CAD build for the part. Positions are in the model's coordinates, mm. Face numbers are marked on the shaded views. Round coordinates to 2 decimals unless told otherwise and drop trailing zeros. Loops run counter-clockwise (first coordinate to the right, second up) from the corner with the lowest first, then second, coordinate; pieces in that order, holes last.
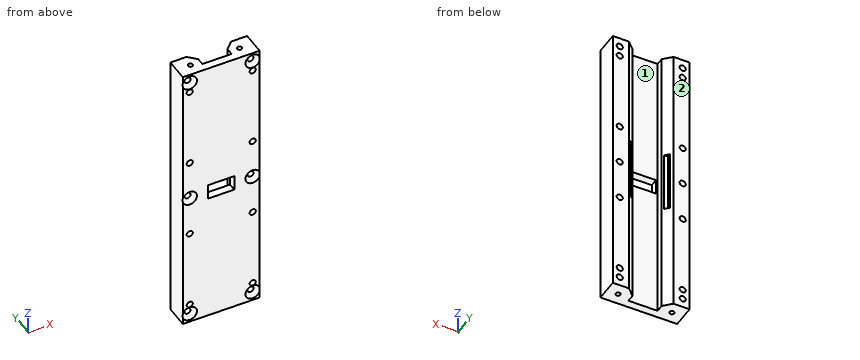
```python
from build123d import *

# Parameters (mm, degrees)
BOSS_EXTRU_1_DEPTH       = 184
ESQUISSE2_R              = 2
ENL_V_MAT_EXTRU_1_DEPTH  = 205.56
ESQUISSE4_R              = 2
ENL_V_MAT_EXTRU_2_DEPTH  = 205.56
CHANFREIN1_SIZE          = 2.7
ESQUISSE6_W              = 26
ESQUISSE6_H              = 40
ENL_V_MAT_EXTRU_3_DEPTH  = 4
ESQUISSE8_W              = 17
ESQUISSE8_H              = 10
ENL_V_MAT_EXTRU_6_DEPTH  = 10
ESQUISSE7_R              = 1.5
ENL_V_MAT_EXTRU_5_DEPTH  = 5
ESQUISSE9_R              = 1.5
ENL_V_MAT_EXTRU_10_DEPTH = 5


with BuildPart() as part:
    # Esquisse1 → Boss.-Extru.1 (new body)
    with BuildSketch(Plane.XY):
        Polygon((0, 0), (50, 0), (50, 15), (39.5, 15), (34.5, 10), (34.5, 5.083005244), (15.5, 5.083005244), (15.5, 10), (10.5, 15), (0, 15), align=None)
    extrude(amount=BOSS_EXTRU_1_DEPTH)

    # Esquisse2 → Enlèv. mat.-Extru.1 (cut)
    with BuildSketch(Plane(origin=(0, 15, 0), x_dir=(-1, 0, 0), z_dir=(0, 1, 0))):
        with Locations(Location((-4.5, 12.78, 0), (0, 0, 90))):
            Circle(ESQUISSE2_R)
        with Locations(Location((-45.5, 12.78, 0), (0, 0, 90))):
            Circle(ESQUISSE2_R)
        with Locations(Location((-4.5, 65.52, 0), (0, 0, 90))):
            Circle(ESQUISSE2_R)
        with Locations(Location((-45.5, 65.52, 0), (0, 0, 90))):
            Circle(ESQUISSE2_R)
        with Locations(Location((-4.5, 118.26, 0), (0, 0, 90))):
            Circle(ESQUISSE2_R)
        with Locations(Location((-45.5, 118.26, 0), (0, 0, 90))):
            Circle(ESQUISSE2_R)
        with Locations(Location((-4.5, 171, 0), (0, 0, 90))):
            Circle(ESQUISSE2_R)
        with Locations(Location((-45.5, 171, 0), (0, 0, 90))):
            Circle(ESQUISSE2_R)
    extrude(amount=-ENL_V_MAT_EXTRU_1_DEPTH, mode=Mode.SUBTRACT)

    # Esquisse4 → Enlèv. mat.-Extru.2 (cut)
    with BuildSketch(Plane(origin=(0, 15, 0), x_dir=(-1, 0, 0), z_dir=(0, 1, 0))):
        with Locations(Location((-4.5, 6, 0), (0, 0, 90))):
            Circle(ESQUISSE4_R)
        with Locations(Location((-45.5, 6, 0), (0, 0, 90))):
            Circle(ESQUISSE4_R)
        with Locations(Location((-45.5, 178, 0), (0, 0, 90))):
            Circle(ESQUISSE4_R)
        with Locations(Location((-4.5, 178, 0), (0, 0, 90))):
            Circle(ESQUISSE4_R)
        with Locations(Location((-4.5, 92, 0), (0, 0, 90))):
            Circle(ESQUISSE4_R)
        with Locations(Location((-45.5, 92, 0), (0, 0, 90))):
            Circle(ESQUISSE4_R)
    extrude(amount=-ENL_V_MAT_EXTRU_2_DEPTH, mode=Mode.SUBTRACT)

    # Chanfrein1
    # the kernel refuses this chamfer: 2.7 mm, written as the material it takes off along each edge
    with BuildSketch(Plane(origin=(4.5, 0, 6), x_dir=(0, 0, 1), z_dir=(-1, 0, 0))) as chanfrein1_piece_1:
        Polygon((2 + CHANFREIN1_SIZE, 0), (2, CHANFREIN1_SIZE), (2, 0), align=None)
    revolve(axis=Axis((4.5, 0, 6), (0, 1, 0)), mode=Mode.SUBTRACT)
    with BuildSketch(Plane(origin=(45.5, 0, 6), x_dir=(0, 0, 1), z_dir=(-1, 0, 0))) as chanfrein1_piece_2:
        Polygon((2 + CHANFREIN1_SIZE, 0), (2, CHANFREIN1_SIZE), (2, 0), align=None)
    revolve(axis=Axis((45.5, 0, 6), (0, 1, 0)), mode=Mode.SUBTRACT)
    with BuildSketch(Plane(origin=(45.5, 0, 178), x_dir=(0, 0, 1), z_dir=(-1, 0, 0))) as chanfrein1_piece_3:
        Polygon((2 + CHANFREIN1_SIZE, 0), (2, CHANFREIN1_SIZE), (2, 0), align=None)
    revolve(axis=Axis((45.5, 0, 178), (0, 1, 0)), mode=Mode.SUBTRACT)
    with BuildSketch(Plane(origin=(4.5, 0, 178), x_dir=(0, 0, 1), z_dir=(-1, 0, 0))) as chanfrein1_piece_4:
        Polygon((2 + CHANFREIN1_SIZE, 0), (2, CHANFREIN1_SIZE), (2, 0), align=None)
    revolve(axis=Axis((4.5, 0, 178), (0, 1, 0)), mode=Mode.SUBTRACT)
    with BuildSketch(Plane(origin=(4.5, 0, 92), x_dir=(0, 0, 1), z_dir=(-1, 0, 0))) as chanfrein1_piece_5:
        Polygon((2 + CHANFREIN1_SIZE, 0), (2, CHANFREIN1_SIZE), (2, 0), align=None)
    revolve(axis=Axis((4.5, 0, 92), (0, 1, 0)), mode=Mode.SUBTRACT)
    with BuildSketch(Plane(origin=(45.5, 0, 92), x_dir=(0, 0, 1), z_dir=(-1, 0, 0))) as chanfrein1_piece_6:
        Polygon((2 + CHANFREIN1_SIZE, 0), (2, CHANFREIN1_SIZE), (2, 0), align=None)
    revolve(axis=Axis((45.5, 0, 92), (0, 1, 0)), mode=Mode.SUBTRACT)

    # Esquisse6 → Enlèv. mat.-Extru.3 (cut)
    with BuildSketch(Plane(origin=(0, 15, 0), x_dir=(1, 0, 0), z_dir=(0, 1, 0))):
        with Locations((25, -92)):
            Rectangle(ESQUISSE6_W, ESQUISSE6_H)
    extrude(amount=-ENL_V_MAT_EXTRU_3_DEPTH, mode=Mode.SUBTRACT)

    # Esquisse8 → Enlèv. mat.-Extru.6 (cut)
    with BuildSketch(Plane(origin=(0, 5.083005244, 0), x_dir=(1, 0, 0), z_dir=(0, 1, 0))):
        with Locations((25, -92)):
            Rectangle(ESQUISSE8_W, ESQUISSE8_H)
    extrude(amount=-ENL_V_MAT_EXTRU_6_DEPTH, mode=Mode.SUBTRACT)

    # Esquisse7 → Enlèv. mat.-Extru.5 (cut)
    with BuildSketch(Plane.XY.offset(184)):
        with Locations((9, 7.5)):
            Circle(ESQUISSE7_R)
        with Locations((41, 7.5)):
            Circle(ESQUISSE7_R)
    extrude(amount=-ENL_V_MAT_EXTRU_5_DEPTH, mode=Mode.SUBTRACT)

    # Esquisse9 → Enlèv. mat.-Extru.10 (cut)
    with BuildSketch(Plane(origin=(0, 0, 0), x_dir=(-1, 0, 0), z_dir=(0, 0, -1))):
        with Locations((-42.5, 7.5)):
            Circle(ESQUISSE9_R)
        with Locations((-7.5, 7.5)):
            Circle(ESQUISSE9_R)
    extrude(amount=-ENL_V_MAT_EXTRU_10_DEPTH, mode=Mode.SUBTRACT)


solid = part.part
```
Item 1: Two-plate mould, pull along X, no slides. Class the marked faces 1 and 2: released by +X, released by -X, zero draft, split by the parting line, or undercut.
Answers follow:
face 1: undercut
face 2: zero draft
Item 2: Cut at A-A, the plane z = 12.78. Give the cut face in (x, y).
Answers follow:
outline: (0, 0) - (2.5, 0) - (2.5, 15) - (0, 15) - close; (6.5, 0) - (43.5, 0) - (43.5, 15) - (39.5, 15) - (34.5, 10) - (34.5, 5.08) - (15.5, 5.08) - (15.5, 10) - (10.5, 15) - (6.5, 15) - close; (47.5, 0) - (50, 0) - (50, 15) - (47.5, 15) - close
Item 3: Flat gauge pins, fed straight in: P1, Ø8, axis at y = 5, z = 81, coming from the -X side; P2, Ø1.2, axis at x = 12.5, z = 87.5, coming from the +Y side; P3, Ø6.5, axis at x = 45.5, z = 178, coming from the -Y side; P4, Ø1.4, axis at x = 43, y = 7.5, coming from the -Z side. Where does each tip first touch, or does it go through?
Answers follow:
P1: stops at x = 0
P2: stops at y = 13.6
P3: stops at y = 1.45
P4: stops at z = 5
Item 4: Cut at B-B, the plane z = 122. Give the cut face in (x, y).
Answers follow:
outline: (0, 0) - (50, 0) - (50, 15) - (39.5, 15) - (34.5, 10) - (34.5, 5.08) - (15.5, 5.08) - (15.5, 10) - (10.5, 15) - (0, 15) - close
Item 5: Probe line 1 (X direction, y = 8.5, z = 12.78); line 2 (X direction, y = 5, z = 13); line 3 (X direction, y = 7.25, z = 102.5). List the from-to ranges inside material, lowest first.
Answers follow:
line 1: x = 0 to 2.5, 6.5 to 15.5, 34.5 to 43.5, 47.5 to 50
line 2: x = 0 to 2.51, 6.49 to 43.51, 47.49 to 50
line 3: x = 0 to 15.5, 34.5 to 50
